from build123d import *

# Parameters (mm, degrees)
BOSS_EXTRUDE1_DEPTH = 80
CUT_EXTRUDE1_DEPTH  = 10
CUT_EXTRUDE2_REACH  = 106.403


with BuildPart() as part:
    # Sketch2 → Boss-Extrude1 (new body)
    with BuildSketch(Plane(origin=(0, 0, 0), x_dir=(0, 0, -1), z_dir=(1, 0, 0))):
        Polygon((0, 0), (0, 30), (-30, 30), (-30, 20), (-60, 0), align=None)
    extrude(amount=BOSS_EXTRUDE1_DEPTH)

    # Sketch3 → Cut-Extrude1 (cut)
    with BuildSketch(Plane(origin=(0, 30, 0), x_dir=(1, 0, 0), z_dir=(0, 1, 0))):
        Polygon((50, 0), (30, 0), (20, -30), (60, -30), align=None)
    extrude(amount=-CUT_EXTRUDE1_DEPTH, mode=Mode.SUBTRACT)

    # Sketch4 → Cut-Extrude2 (cut, up to next)
    with BuildSketch(Plane.XZ, mode=Mode.PRIVATE) as cut_extrude2_sk1:
        Polygon((60, 60), (20, 60), (30, 40), (50, 40), align=None)
    cut_extrude2_tool1 = extrude(cut_extrude2_sk1.sketch, amount=-CUT_EXTRUDE2_REACH, mode=Mode.PRIVATE) & part.part
    add(cut_extrude2_tool1.solids().sort_by_distance((40, 0, 51.111111))[0], mode=Mode.SUBTRACT)


solid = part.part
Can you work these out from the model? Positions are in its coordinate system, mm. A direction names the side the tool comes from. Coordinates: 2 decimals unless noted, no trailing zeros. Write each loop counter-clockwise with the first axis right and the second up, starting at its lowest first coordinate (ties: lowest second). Pieces come first, ordered by that corner, then holes. Notation, with made-up numbers: (22.5, 30.25) -> (31.5, 30.25) arc R25 ccw to (31.5, 55.25) -> close; hole circle Ø9 at (61.25, 72.5). An arc over 180 degrees is marked (long way). Write each question's results on one line, items separated by ' | '. Start each with the question number.
Item 1: On a 3-axis mill with a long thin cutter (end or side, diameter ignored), from which of +Z, -Z, +X, -X, +Y, -Y can I reach the whole of each face in a straight line? I mean faces 1 (the flat face through (10, 25, 30)), 2 (the flat face through (39, 15, 0)), 3 (the flat face through (27, 4, 46)), 4 (the flat face through (68, 30, 15)), 5 (the flat face through (40, 20, 18)). Say none if no direction works.
Item 2: I'm going to push flat-ended pins straight in: P1, Ø5, axis at x = 67, y = 25, coming from the +Z side; P2, Ø9, axis at x = 38.5, z = 21.5, coming from the +Y side; P3, Ø10, axis at x = 32.5, y = 10, coming from the +Z side. Where does each tip first touch, or does it pass through?
Item 3: If we section it at D-D, the plane y = 12: Write out the boundary of the cut face in (x, z).
Item 4: If we section it at A-A, the plane y = 24: Write out the boundary of the cut face in (x, z), and give its area (3 significant figures).
Item 5: If we section it at C-C, the plane x = 51: Write out the boundary of the cut face in (y, z).
Item 6: Please list where these lines run through material, in increasing order: probe 1 along Y at (x, z) = (44.5, 12.5); probe 2 along X at (y, z) = (3, 50.5); probe 3 along Z at (x, y) = (31, 11.5).
Item 7: If we section it at B-B, the plane z = 56.5: Write out the boundary of the cut face in (x, y).
Item 8: Thinking about a two-plate mould opening in X: for faces 6 (the flat face through (70, 25, 30)), 7 (the flat face through (0, 12, 24)), 8 (the flat face through (55, 25, 15)), 9 (the flat face through (80, 12, 24)), which applies, released by +X, released by -X, zero draft, split by the parting line, or undercut?
Answer block:
1) face 1: +Z, +X, -X, +Y | face 2: -Z, +X, -X, +Y, -Y | face 3: +Z, +Y, -Y | face 4: +Z, -Z, +X, -X, +Y | face 5: +Z, +Y
2) P1: z = 30 | P2: y = 20 | P3: z = 45
3) outline: (0, 0) -> (80, 0) -> (80, 42) -> (51, 42) -> (50, 40) -> (30, 40) -> (29, 42) -> (0, 42) -> close
4) outline: (0, 0) -> (30, 0) -> (20, 30) -> (0, 30) -> close; (50, 0) -> (80, 0) -> (80, 30) -> (60, 30) -> close | area: 1,500 mm²
5) outline: (0, 0) -> (30, 0) -> (30, 3) -> (20, 3) -> (20, 30) -> (12, 42) -> (0, 42) -> close
6) probe 1: 0 to 20 | probe 2: 0 to 24.75, 55.25 to 80 | probe 3: 0 to 40
7) outline: (0, 0) -> (21.75, 0) -> (21.75, 2.33) -> (0, 2.33) -> close; (58.25, 0) -> (80, 0) -> (80, 2.33) -> (58.25, 2.33) -> close
8) face 6: zero draft | face 7: released by -X | face 8: undercut | face 9: released by +X
